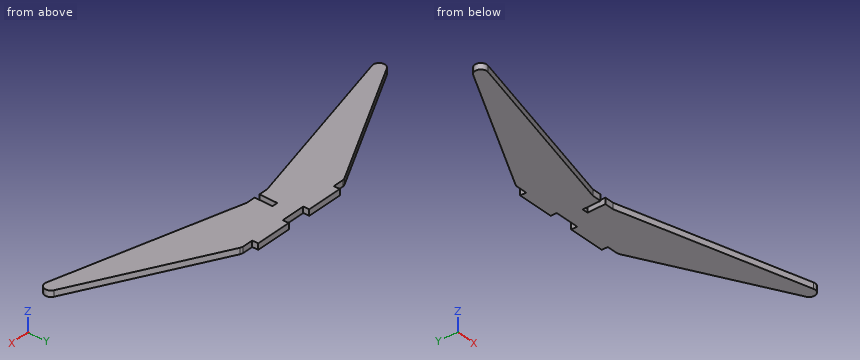
```python
from build123d import *

# Parameters (mm, degrees)
BOSS_EXTRUDE1_DEPTH = 3.175


with BuildPart() as part:
    # Sketch1 → Boss-Extrude1 (new body)
    with BuildSketch(Plane.XY):
        with BuildLine():
            Line((25.4, 0), (30.968022768, 0))
            ThreePointArc((30.968022768, 0), (31.727309935, -0.092126666), (32.442533736, -0.363160318))
            Line((32.442533736, -0.363160318), (104.164919452, -37.973926384))
            ThreePointArc((104.164919452, -37.973926384), (105.652252875, -41.929489282), (101.892440564, -43.858854448))
            Line((101.892440564, -43.858854448), (6.35, -19.05))
            Line((6.35, -19.05), (1.4859, -19.05))
            Line((1.4859, -19.05), (1.4859, -9.6266))
            Line((1.4859, -9.6266), (-1.4859, -9.6266))
            Line((-1.4859, -9.6266), (-1.4859, -19.05))
            Line((-1.4859, -19.05), (-6.35, -19.05))
            Line((-6.35, -19.05), (-100.721752752, -43.884671777))
            ThreePointArc((-100.721752752, -43.884671777), (-104.48570891, -41.973107935), (-103.023886624, -38.012739532))
            Line((-103.023886624, -38.012739532), (-32.450367647, -0.373529412))
            ThreePointArc((-32.450367647, -0.373529412), (-31.726300609, -0.094797562), (-30.95625, 0))
            Line((-30.95625, 0), (-25.4, 0))
            Line((-25.4, 0), (-25.399999646, 3.174999957))
            Line((-25.399999646, 3.174999957), (-6.349999646, 3.174999957))
            Line((-6.349999646, 3.174999957), (-6.35, 0))
            Line((-6.35, 0), (6.35, 0))
            Line((6.35, 0), (6.350000354, 3.174999957))
            Line((6.350000354, 3.174999957), (25.400000354, 3.174999957))
            Line((25.400000354, 3.174999957), (25.4, 0))
        make_face()
    extrude(amount=BOSS_EXTRUDE1_DEPTH)


solid = part.part
```
Model file for the job. Use its own axes, mm. Round coordinates to 2 decimals unless told otherwise and drop trailing zeros. Write each loop counter-clockwise with the first axis right and the second up, starting at its lowest first coordinate (ties: lowest second). Pieces come first, ordered by that corner, then holes. Notation, with made-up numbers: (-3, 63) - (54, 63) arc R10 ccw to (54, 71) - close; hole circle Ø6 at (83, 63). An arc over 180 degrees is marked (long way). One line per item, written item: value.
(1) Drop flat-ended pins along their axis: P1, Ø1.6, axis at y = 1.5, z = 1, coming from the -X side; P2, Ø1, axis at x = -4, z = 1.5, coming from the -Y side; P3, Ø1.6, axis at y = 2, z = 2, coming from the +X side. Give the stop position or say it passes through.
Values follow:
P1: stops at x = -25.4
P2: stops at y = -19.05
P3: stops at x = 25.4
(2) Cut at C-C, the plane x = -65. Give the cut face in (y, z) (3 decimals).
Values follow:
outline: (-34.484, 0) - (-17.733, 0) - (-17.733, 3.175) - (-34.484, 3.175) - close
(3) Wall check: probe 1 along X at (y, z) = (1.5, 1.8); probe 2 along X at (y, z) = (-18, 2.7); probe 3 along X at (y, z) = (-4.5, 2.55). Give the ranges that are in metal, low to high.
Values follow:
probe 1: x = -25.4 to -6.35, 6.35 to 25.4
probe 2: x = -65.5 to -1.49, 1.49 to 66.08
probe 3: x = -40.19 to 40.33
(4) Cut at D-D, the plane y = -5. Give the cut face in (x, z) (3 decimals), plus the area to 3 significant figures.
Values follow:
outline: (-41.125, 0) - (41.285, 0) - (41.285, 3.175) - (-41.125, 3.175) - close
area: 262 mm²
(5) Cut at B-B, the plane y = -26. Give the cut face in (x, z) (3 decimals).
Values follow:
outline: (-80.5, 0) - (-32.76, 0) - (-32.76, 3.175) - (-80.5, 3.175) - close; (33.115, 0) - (81.331, 0) - (81.331, 3.175) - (33.115, 3.175) - close
(6) Cut at A-A, the plane z = 1.7. Give the cut face in (x, y) (3 decimals).
Values follow:
outline: (-103.024, -38.013) arc R3.175 ccw to (-100.722, -43.885) - (-6.35, -19.05) - (-1.486, -19.05) - (-1.486, -9.627) - (1.486, -9.627) - (1.486, -19.05) - (6.35, -19.05) - (101.892, -43.859) arc R3.175 ccw to (104.165, -37.974) - (32.443, -0.363) arc R3.175 ccw to (30.968, 0) - (25.4, 0) - (25.4, 3.175) - (6.35, 3.175) - (6.35, 0) - (-6.35, 0) - (-6.35, 3.175) - (-25.4, 3.175) - (-25.4, 0) - (-30.956, 0) arc R3.175 ccw to (-32.45, -0.374) - close
